Part model, mm, in its own coordinate system. A direction names the side the tool comes from. Give positions to 0.01 mm unless a question says otherwise; leave off trailing zeros. Loops run counter-clockwise (first coordinate to the right, second up) from the corner with the lowest first, then second, coordinate; pieces in that order, holes last. Notation, with made-up numbers: M -33.75,12 L 7.25,12 A26 ccw 7.25,34 Z; hole C 4.5,76 d4. An arc over 180 degrees is marked long. Put each result on its own line as item: value. Start each with the question number.
```python
from build123d import *

# Parameters (mm, degrees)
SKETCH_2_R           = 20
SKETCH_2_R_2         = 17
EXTRUDE_1_DEPTH      = 45
EXTRUDE_2_REACH      = 79.621
EXTRUDE_2_END_RADIUS = 20
SKETCH_3_R           = 10


with BuildPart() as part:
    # 草图2 → 凸台-拉伸1 (new body)
    with BuildSketch(Plane(origin=(0, 0, 0), x_dir=(1, 0, 0), z_dir=(0, 1, 0))):
        with Locations(Location((0, 0, 0), (0, 0, 90))):
            Circle(SKETCH_2_R)
        with Locations(Location((0, 0, 0), (0, 0, 90))):
            Circle(SKETCH_2_R_2, mode=Mode.SUBTRACT)
    extrude(amount=EXTRUDE_1_DEPTH)

    # 凸台-拉伸2: up to this cylinder (the profile starts outside it)
    extrude_2_end = Plane(origin=(0, 22.5, 0), z_dir=(0, -1, 0)) * Cylinder(EXTRUDE_2_END_RADIUS, 200.242, mode=Mode.PRIVATE)
    # 草图3 → 凸台-拉伸2 (add, up to the surface)
    with BuildSketch(Plane.XY.offset(40), mode=Mode.PRIVATE) as extrude_2_sk1:
        with Locations((0, 22.5)):
            Circle(SKETCH_3_R)
    extrude_2_tool1 = extrude(extrude_2_sk1.sketch, amount=-EXTRUDE_2_REACH, mode=Mode.PRIVATE) - extrude_2_end
    extrude_2 = extrude_2_tool1.solids().sort_by_distance((0, 22.5, 40))[0]
    add(extrude_2)

    # 镜向2: 凸台-拉伸2 across plane
    add(extrude_2.mirror(Plane.XY))


solid = part.part
```
1) Band-saw the part on A-A on z = 0. Give the cut face in (x, y), then the cut area to 3 significant figures.
2) Band-saw the part on C-C on y = 22.5. Give the cut face in (x, z).
3) Mould opens along X. For faces 3 (the cylindrical face through (-16.855, 22.185, 2.213)), 4 (the cylindrical face through (-9.99, 22.94, -28.82)), 5 (the flat face through (15, 0, 9)) say: +X half, -X half, draft (parallel to the pull), parting line (faces both ways), or undercut.
4) Which spindle directions (+Z, -Z, +X, -X, +Y, -Y) get a long thin tool onto all of the face, cutting with end or side? Do faces 1 (the flat face through (0, 23, 40)), 2 (the cylindrical face through (-9.99, 22.94, 28.82)). Say none if no direction does.
5) Pin check, flat tips, straight feed: pin 1 Ø3 at (x, z) = (-4, -13.5) entering from +Y; pin 2 Ø1 at (x, y) = (-14, 20.5) entering from +Z; pin 3 Ø6 at (x, y) = (-15, 26) entering from -Z. Stop position of each tip, or through.
6) Band-saw the part on D-D on x = -15.5. Give the cut face in (y, z).
7) Wall check: L1, parallel to X at y = 26, z = 0; L2, parallel to X at y = 7, z = -15.5; L3, parallel to Z at x = 4, y = 21. Give the ranges that are in metal, low to high.
8) Band-saw the part on B-B on x = 0. Give the cut face in (y, z), then the cut area to 3 significant figures.
Evaluation:
1. outline: M -20,0 L -17,0 L -17,45 L -20,45 Z; M 17,0 L 20,0 L 20,45 L 17,45 Z
1. area: 270 mm2
2. outline: M -10,-40 L 10,-40 L 10,-17.32 A20 ccw 10,17.32 L 10,40 L -10,40 L -10,17.32 A20 ccw -10,-17.32 Z; hole C 0,0 d34
3. face 3: undercut
3. face 4: parting line
3. face 5: draft
4. face 1: +Z, +X, -X, +Y, -Y
4. face 2: +Z
5. pin 1: through
5. pin 2: z = 14.76
5. pin 3: z = -16
6. outline: M 0,-12.64 L 45,-12.64 L 45,-6.98 L 0,-6.98 Z; M 0,6.98 L 45,6.98 L 45,12.64 L 0,12.64 Z
7. L1: -20 to -17, 17 to 20
7. L2: -12.64 to -6.98, 6.98 to 12.64
7. L3: -40 to -16.52, 16.52 to 40
8. outline: M 0,-20 L 12.5,-20 L 12.5,-40 L 32.5,-40 L 32.5,-20 L 45,-20 L 45,-17 L 0,-17 Z; M 0,17 L 45,17 L 45,20 L 32.5,20 L 32.5,40 L 12.5,40 L 12.5,20 L 0,20 Z
8. area: 1,070 mm2
